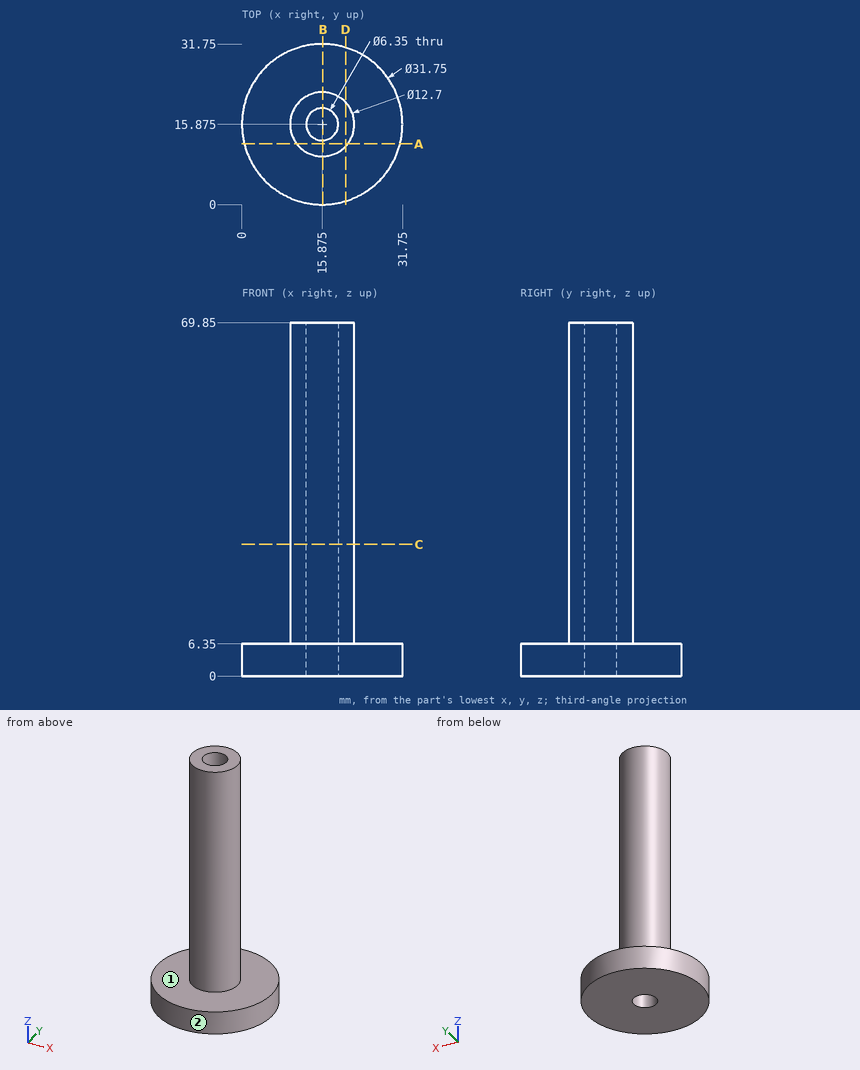
Can you work these out from the drawing? Everything is in mm from the part's minimum corner. A direction names the side the tool comes from. Coordinates: 2 decimals unless noted, no trailing zeros. Loops run counter-clockwise (first coordinate to the right, second up) from the corner with the lowest first, then second, coordinate; pieces in that order, holes last.
1) Imagine slicing it at A-A (y = 12). List the corners of the cut face in (x, z) for me.
Reported:
outline: (0.48, 0) - (31.27, 0) - (31.27, 6.35) - (20.91, 6.35) - (20.91, 69.85) - (10.84, 69.85) - (10.84, 6.35) - (0.48, 6.35) - close
2) Please list where these lines run through material, in increasing order: line 1 along Y through (x, z) = (16, 34.5); line 2 along X through (y, z) = (15.5, 50); line 3 along Z through (x, y) = (20, 9.5).
Reported:
line 1: y = 9.53 to 12.7, 19.05 to 22.22
line 2: x = 9.54 to 12.72, 19.03 to 22.21
line 3: z = 0 to 6.35
3) Imagine slicing it at B-B (x = 16). List the corners of the cut face in (y, z) for me.
Reported:
outline: (0, 0) - (12.7, 0) - (12.7, 69.85) - (9.53, 69.85) - (9.53, 6.35) - (0, 6.35) - close; (19.05, 0) - (31.75, 0) - (31.75, 6.35) - (22.22, 6.35) - (22.22, 69.85) - (19.05, 69.85) - close
4) Which directions (+Z, -Z, +X, -X, +Y, -Y) give clear straight access to the entire face, cutting with the end or side of a thin tool? Please do the marked faces 1 and 2.
Reported:
face 1: +Z
face 2: +Z, -Z
5) Imagine slicing it at C-C (z = 26). List the corners of the cut face in (x, y) for me (3 decimals).
Reported:
outline: circle Ø12.7 at (15.875, 15.875); hole circle Ø6.35 at (15.875, 15.875)
6) Will these pins go through, and if not, where does the flat tip stop? pin 1 Ø5 at (y, z) = (14, 52.5) entering from -X (3 decimals); pin 2 Ø5 at (x, z) = (12.5, 61.5) entering from -Y; pin 3 Ø10 at (x, z) = (10.5, 41.5) entering from +Y; pin 4 Ø5 at (x, y) = (15.875, 15.875) entering from -Z.
Reported:
pin 1: stops at x = 9.525
pin 2: stops at y = 9.59
pin 3: stops at y = 22.21
pin 4: passes through
7) Imagine slicing it at D-D (x = 20.5). List the corners of the cut face in (y, z) for me.
Reported:
outline: (0.69, 0) - (31.06, 0) - (31.06, 6.35) - (20.23, 6.35) - (20.23, 69.85) - (11.52, 69.85) - (11.52, 6.35) - (0.69, 6.35) - close
